from build123d import *

# Parameters (mm, degrees)
F0_R            = 61.184507213
F1_DEPTH        = 25
F2_R            = 14.1604507034
F3_DEPTH        = 25
F5_DEPTH        = 25
F5_COPIES_COUNT = 12


# Not quite as in the source:
# - a pattern or mirror of a feature is missing from the dataset's text; its kind, count and spacing are read off the source's solid


with BuildPart() as f1:
    # F0 (on Front) → F1 (new body)
    with BuildSketch(Plane.XZ):
        Circle(F0_R)
    extrude(amount=F1_DEPTH)

    # F2 (on face) → F3 (cut)
    with BuildSketch(Plane.XZ.offset(25)):
        Circle(F2_R)
    extrude(amount=-F3_DEPTH, mode=Mode.SUBTRACT)

    # F4 (on Front) → F5 (join)
    with BuildSketch(Plane.XZ):
        with BuildLine():
            Line((0, 80), (-8.1378884566, 60.6408995181))
            ThreePointArc((-8.1378884566, 60.6408995181), (0, 61.184507213), (8.1378884566, 60.6408995181))
            Line((8.1378884566, 60.6408995181), (0, 80))
        make_face()
    f5 = extrude(amount=F5_DEPTH)

    # F5_copies: F5 ×12 about axis
    f5_copies_axis = Axis((0, 0, 0), (0, 1, 0))
    for i in range(1, F5_COPIES_COUNT):
        add(f5.rotate(f5_copies_axis, i * 360 / F5_COPIES_COUNT))


solid = f1.part
Input: part model. Units: mm. Frame: model coordinates. A direction names the side the tool comes from. Give positions to 0.01 mm unless a question says otherwise; leave off trailing zeros. Order: outer loops, then holes, each group sorted by start corner. A loop starts at its lowest first (then second) coordinate and runs counter-clockwise, first axis right, second up. Notation, with made-up numbers: (0.5, 74) - (39.5, 74) arc R25 ccw to (39.5, 109) - close; hole circle Ø7 at (-26, -28). An arc over 180 degrees is marked (long way). Answer as a JSON object with one key per item and string values. Group by question number.
Q1. Mould query, pull axis Z, two halves, no side actions, for faces 5 (the face through (-38.666, -12.325, -58.719)), 6 (the face through (15.94, -12.32, 59.07)), 7 (the face through (17, -25, 1)), 8 (the face through (-43.19, -12.32, 43.34)). Classes: pulls with the +Z half, pulls with the -Z half, needs draft (parallel to the pull), parting line crosses it, or undercut.
Q2. First-contact query: pin 1 Ø1 at (x, y) = (-23.5, -16) entering from +Z; pin 2 Ø4 at (x, z) = (-8, -43) entering from +Y; pin 3 Ø12 at (y, z) = (-12.5, -21) entering from -X; pin 4 Ø3 at (x, y) = (12, -11.5) entering from +Z. Flat tips, straight axial feed; report the tip coordinate or a pass-through.
Q3. Cut plane D-D, the plane x = -27. Output: boundary loops of the cut face in (y, z).
Q4. Cut plane A-A, the plane x = -5. Output: boundary loops of the cut face in (y, z), then the cut area to 3 significant figures.
Q5. Line query: probe 1 along Z at (x, y) = (-66, -15.5); probe 2 along X at (y, z) = (-2.5, 63); probe 3 along X at (y, z) = (-3.75, 64). Output: solid intervals per line, ascending.
Q6. Set-up query: faces 1 (the face through (43.19, -12.32, -43.34)), 2 (the face through (-59.07, -12.32, 15.94)), 3 (the face through (-31.519, -12.325, 62.845)), 4 (the face through (-15.94, -12.32, -59.07)). Return all of +Z, -Z, +X, -X, +Y, -Y with unobstructed straight access to the full face (end or side cutting, diameter ignored); none if empty.
Q7. Cut plane B-B, the plane x = 67. Output: boundary loops of the cut face in (y, z).
Q8. Cut plane C-C, the plane z = 32.5. Output: boundary loops of the cut face in (x, y), then the cut area to 3 significant figures.
Results:
{
 "1": {"face 5": "undercut", "face 6": "pulls with the +Z half", "face 7": "needs draft", "face 8": "undercut"},
 "2": {"pin 1": "z = 57.14", "pin 2": "y = 0", "pin 3": "x = -59.41", "pin 4": "z = 60.28"},
 "3": {"outline": "(-25, -59.41) - (0, -59.41) - (0, 59.41) - (-25, 59.41) - close"},
 "4": {"outline": "(-25, -68.11) - (0, -68.11) - (0, -13.25) - (-25, -13.25) - close; (-25, 13.25) - (0, 13.25) - (0, 68.11) - (-25, 68.11) - close", "area": "2,740 mm^2"},
 "5": {"probe 1": "-39.59 to -35.68, -5.89 to 5.89, 35.68 to 39.59", "probe 2": "-39.21 to -31.72, -7.15 to 7.15, 31.72 to 39.21", "probe 3": "-39.33 to -33.04, -6.73 to 6.73, 33.04 to 39.33"},
 "6": {"face 1": "+Y, -Y", "face 2": "-X, +Y, -Y", "face 3": "+Z, +Y, -Y", "face 4": "-Z, +Y, -Y"},
 "7": {"outline": "(-25, -39.71) - (0, -39.71) - (0, -36.99) - (-25, -36.99) - close; (-25, -5.46) - (0, -5.46) - (0, 5.46) - (-25, 5.46) - close; (-25, 36.99) - (0, 36.99) - (0, 39.71) - (-25, 39.71) - close"},
 "8": {"outline": "(-63.59, -25) - (63.59, -25) - (63.59, 0) - (-63.59, 0) - close", "area": "3,180 mm^2"}
}
